Check sheet for the modelled part. Datum: model origin and axes. Units: mm. A direction names the side the tool comes from. Round coordinates to 2 decimals unless told otherwise and drop trailing zeros. Order: outer loops, then holes, each group sorted by start corner. A loop starts at its lowest first (then second) coordinate and runs counter-clockwise, first axis right, second up.
(1) Mould release check, pull along Y, two halves, no side actions. Record for faces 1 (the cylindrical face through (31.4, -80, 16.7)), 2 (the flat face through (62, -33, 16)), 3 (the flat face through (87.4, -44.7, 19.3)), 4 (the flat face through (28.6, -45, 32.3)): released by +Y, released by -Y, zero draft, split by the parting line, or undercut.
(2) Sectioned sample at C-C, the plane y = -7. Enter the section's corners in (x, z).
(3) Sectioned sample at A-A, the plane x = 53.5. Enter the section's corners in (y, z) (1 decimal), and give its area (3 significant figures).
(4) Sectioned sample at D-D, the plane x = 80. Enter the section's corners in (y, z).
(5) Thickness scan on probe 1 along Y at (x, z) = (5.5, 19); probe 2 along X at (y, z) = (-23.5, 14); probe 3 along Z at (x, y) = (13, -53). Record the ranges inside material, lowest first.
(6) Sectioned sample at B-B, the plane y = -65. Enter the section's corners in (x, z), and give its area (3 significant figures).
(7) Tool access check on faces 5 (the flat face through (31, -62, 1)), 6 (the flat face through (86.148, -44.694, 11.522)), 7 (the flat face through (62.667, -75, 24)), 8 (the flat face through (78.763, -44.694, 8.687)). Record the directions out of +Z, -Z, +X, -X, +Y, -Y that give a thin tool (end or side, any length) a straight path to the whole face; none if there is none.
(8) Depth check by flat-ended pin: pin 1 (1 mm diameter, centred on x = 58, z = 27.5, fed in from -Y); pin 2 (2 mm diameter, centred on y = -48, z = 20.5, fed in from +X); pin 3 (0.6 mm diameter, centred on x = 63.5, y = -18, fed in from -Z). Enter the tip coordinate at first touch or a pass-through.
```python
from build123d import *

# Parameters (mm, degrees)
CROQUIS1_W               = 62
CROQUIS1_H               = 45
SALIENTE_EXTRUIR1_DEPTH  = 33
CROQUIS2_W               = 25.463929144
CROQUIS2_H               = 24.410779192
SALIENTE_EXTRUIR2_DEPTH  = 2
CROQUIS3_W               = 24.282059014
CROQUIS3_H               = 23.443794542
SALIENTE_EXTRUIR3_DEPTH  = 26
CROQUIS5_W               = 41.33364391
CROQUIS5_H               = 31
SALIENTE_EXTRUIR5_DEPTH  = 35
CROQUIS6_W               = 31
CROQUIS6_H               = 30
SALIENTE_EXTRUIR6_DEPTH  = 11
CROQUIS7_W               = 31
CROQUIS7_H               = 30
SALIENTE_EXTRUIR7_DEPTH  = 11
CORTAR_EXTRUIR1_DEPTH    = 11
CORTAR_EXTRUIR2_DEPTH    = 52.33364391
CORTAR_EXTRUIR3_START    = -11
CORTAR_EXTRUIR3_DEPTH    = 11
CROQUIS17_R              = 9
SALIENTE_EXTRUIR8_DEPTH  = 16
CROQUIS18_R              = 5.625205596
SALIENTE_EXTRUIR9_DEPTH  = 2
SALIENTE_EXTRUIR10_DEPTH = 4
CROQUIS20_R              = 11.5
CORTAR_EXTRUIR6_DEPTH    = 63.33364391


with BuildPart() as part:
    # Croquis1 → Saliente-Extruir1 (new body)
    with BuildSketch(Plane.XY):
        with Locations((31, -22.5)):
            Rectangle(CROQUIS1_W, CROQUIS1_H)
    extrude(amount=SALIENTE_EXTRUIR1_DEPTH)

    # Croquis2 → Saliente-Extruir2 (add)
    with BuildSketch(Plane(origin=(62, 0, 0), x_dir=(0, 0, -1), z_dir=(1, 0, 0))):
        with Locations((-16.5, -13)):
            Rectangle(CROQUIS2_W, CROQUIS2_H)
    extrude(amount=SALIENTE_EXTRUIR2_DEPTH)

    # Croquis3 → Saliente-Extruir3 (add)
    with BuildSketch(Plane(origin=(64, 0, 0), x_dir=(0, 0, -1), z_dir=(1, 0, 0))):
        with Locations((-16.5, -13)):
            Rectangle(CROQUIS3_W, CROQUIS3_H)
    extrude(amount=SALIENTE_EXTRUIR3_DEPTH)

    # Croquis5 → Saliente-Extruir5 (add)
    with BuildSketch(Plane.XZ.offset(45)):
        with Locations((31, 16.5)):
            Rectangle(CROQUIS5_W, CROQUIS5_H)
    extrude(amount=SALIENTE_EXTRUIR5_DEPTH)

    # Croquis6 → Saliente-Extruir6 (add)
    with BuildSketch(Plane(origin=(51.666821955, 0, 0), x_dir=(0, 0, -1), z_dir=(1, 0, 0))):
        with Locations((-16.5, -65)):
            Rectangle(CROQUIS6_W, CROQUIS6_H)
    extrude(amount=SALIENTE_EXTRUIR6_DEPTH)

    # Croquis7 → Saliente-Extruir7 (add)
    with BuildSketch(Plane.ZY.offset(-10.333178045)):
        with Locations((16.5, -65)):
            Rectangle(CROQUIS7_W, CROQUIS7_H)
    extrude(amount=SALIENTE_EXTRUIR7_DEPTH)

    # Croquis8 → Cortar-Extruir1 (cut)
    with BuildSketch(Plane(origin=(62.666821955, 0, 0), x_dir=(0, 0, -1), z_dir=(1, 0, 0))):
        with BuildLine():
            Line((-32, -80), (-32, -78))
            ThreePointArc((-32, -78), (-16.5, -80), (-1, -78))
            Line((-1, -78), (0.928970142, -80.475031326))
            Line((0.928970142, -80.475031326), (-0.274135128, -81.99339903))
            Line((-0.274135128, -81.99339903), (-8.695872018, -84.279445288))
            Line((-8.695872018, -84.279445288), (-24.986567701, -83.98679806))
            Line((-24.986567701, -83.98679806), (-32, -80))
        make_face()
        with BuildLine():
            Line((-32, -52), (-33.723093641, -49.93126323))
            Line((-33.723093641, -49.93126323), (-34.225322301, -47.788491738))
            Line((-34.225322301, -47.788491738), (-30.90530883, -47.311645213))
            Line((-30.90530883, -47.311645213), (-17.951536569, -46.72536261))
            Line((-17.951536569, -46.72536261), (-10.133210988, -47.311645213))
            Line((-10.133210988, -47.311645213), (0, -48.071517035))
            Line((0, -48.071517035), (0, -49))
            Line((0, -49), (-1, -52))
            ThreePointArc((-1, -52), (-16.5, -50), (-32, -52))
        make_face()
    extrude(amount=-CORTAR_EXTRUIR1_DEPTH, mode=Mode.SUBTRACT)

    # Croquis9 → Cortar-Extruir2 (cut)
    with BuildSketch(Plane(origin=(51.666821955, 0, 0), x_dir=(0, 0, -1), z_dir=(1, 0, 0))):
        with BuildLine():
            Line((-32, -78), (-33.497607454, -80))
            Line((-33.497607454, -80), (-33.497607454, -82.886987671))
            Line((-33.497607454, -82.886987671), (-32, -84.384595125))
            Line((-32, -84.384595125), (-22.575228316, -85.712467989))
            Line((-22.575228316, -85.712467989), (-14.351815451, -85.712467989))
            Line((-14.351815451, -85.712467989), (-8.532169423, -85.048531557))
            Line((-8.532169423, -85.048531557), (-1, -84.384595125))
            Line((-1, -84.384595125), (0.769167017, -82.615428108))
            Line((0.769167017, -82.615428108), (1.462440059, -80.483220833))
            Line((1.462440059, -80.483220833), (1.462440059, -79))
            Line((1.462440059, -79), (-1, -78))
            ThreePointArc((-1, -78), (-16.5, -80), (-32, -78))
        make_face()
    extrude(amount=-CORTAR_EXTRUIR2_DEPTH, mode=Mode.SUBTRACT)

    # Croquis10 → Cortar-Extruir3 (cut)
    with BuildSketch(Plane.ZY.offset(0.666821955).offset(CORTAR_EXTRUIR3_START)):
        with BuildLine():
            Line((32, -52), (34.151499122, -49.263012271))
            Line((34.151499122, -49.263012271), (33.075749561, -47.196000203))
            Line((33.075749561, -47.196000203), (22.583484216, -46.688313029))
            Line((22.583484216, -46.688313029), (7.099025391, -47.631160639))
            Line((7.099025391, -47.631160639), (-1.096496141, -48.229506237))
            Line((-1.096496141, -48.229506237), (1, -52))
            ThreePointArc((1, -52), (16.5, -50), (32, -52))
        make_face()
    extrude(amount=CORTAR_EXTRUIR3_DEPTH, mode=Mode.SUBTRACT)

    # Croquis17 → Saliente-Extruir8 (add)
    with BuildSketch(Plane.XZ.offset(24.721897271)):
        with Locations(Location((80, 16.5, 0), (0, 0, 90))):
            Circle(CROQUIS17_R)
    extrude(amount=SALIENTE_EXTRUIR8_DEPTH)

    # Croquis18 → Saliente-Extruir9 (add)
    with BuildSketch(Plane.XZ.offset(40.721897271)):
        with Locations((80, 16.5)):
            Circle(CROQUIS18_R)
    extrude(amount=SALIENTE_EXTRUIR9_DEPTH)

    # Croquis19 → Saliente-Extruir10 (add)
    with BuildSketch(Plane.XZ.offset(42.721897271)):
        Polygon((89.032919524, 15.145062071), (85.689870429, 23.645268814), (76.656950905, 25.000206743), (70.967080476, 17.854937929), (74.310129571, 9.354731186), (83.343049095, 7.999793257), align=None)
    extrude(amount=SALIENTE_EXTRUIR10_DEPTH)

    # Croquis20 → Cortar-Extruir6 (cut)
    with BuildSketch(Plane(origin=(62.666821955, 0, 0), x_dir=(0, 0, -1), z_dir=(1, 0, 0))):
        with Locations((-16.5, -65)):
            Circle(CROQUIS20_R)
    extrude(amount=-CORTAR_EXTRUIR6_DEPTH, mode=Mode.SUBTRACT)


solid = part.part
```
Derived:
1. face 1: released by -Y
1. face 2: undercut
1. face 3: zero draft
1. face 4: undercut
2. outline: (0, 0) - (62, 0) - (62, 3.77) - (64, 3.77) - (64, 4.36) - (90, 4.36) - (90, 28.64) - (64, 28.64) - (64, 29.23) - (62, 29.23) - (62, 33) - (0, 33) - close
3. outline: (-78, 1) - (-52, 1) arc R61.1 ccw to (-52, 32) - (-78, 32) arc R61.1 ccw to start; (-45, 0) - (0, 0) - (0, 33) - (-45, 33) - close; hole circle Ø23 at (-65, 16.5)
3. area: 1,960 mm2
4. outline: (-46.72, 8.5) - (-42.72, 8.5) - (-42.72, 10.87) - (-40.72, 10.87) - (-40.72, 7.5) - (-24.72, 7.5) - (-24.72, 4.36) - (-1.28, 4.36) - (-1.28, 28.64) - (-24.72, 28.64) - (-24.72, 25.5) - (-40.72, 25.5) - (-40.72, 22.13) - (-42.72, 22.13) - (-42.72, 24.5) - (-46.72, 24.5) - close
5. probe 1: y = -79.95 to -76.22, -53.78 to -50.05, -45 to 0
5. probe 2: x = 0 to 90
5. probe 3: z = 1 to 32
6. outline: (-0.67, 1) - (62.67, 1) - (62.67, 5) - (-0.67, 5) - close; (-0.67, 28) - (62.67, 28) - (62.67, 32) - (-0.67, 32) - close
6. area: 507 mm2
7. face 5: -Z, +X, -X, -Y
7. face 6: -Z, +X, -Y
7. face 7: +Z, -Z, +X, -Y
7. face 8: -Z, -Y
8. pin 1: stops at y = -79.09
8. pin 2: stops at x = 51.67
8. pin 3: stops at z = 3.77
